Could you check a few things on this model? Use its own coordinates, in mm. A direction names the side the tool comes from. Round coordinates to 2 decimals unless told otherwise and drop trailing zeros. Loops run counter-clockwise (first coordinate to the right, second up) from the corner with the lowest first, then second, coordinate; pieces in that order, holes last. Notation, with made-up numbers: (-3, 66.5) - (32, 66.5) arc R37 ccw to (32, 104.5) - close; hole circle Ø5 at (50.25, -21). An arc over 180 degrees is marked (long way). Put each result on its own line as item: value. Start each with the question number.
from build123d import *

# Parameters (mm, degrees)
CROQUIS1_R              = 13
CROQUIS1_R_2            = 6
SALIENTE_EXTRUIR1_DEPTH = 10
CROQUIS2_W              = 30
CROQUIS2_H              = 15
SALIENTE_EXTRUIR2_DEPTH = 5
CROQUIS3_W              = 30
CROQUIS3_H              = 5
SALIENTE_EXTRUIR3_DEPTH = 20
CROQUIS4_R              = 5
CORTAR_EXTRUIR1_DEPTH   = 20
REDONDEO1_R             = 1
REDONDEO2_R             = 1
REDONDEO3_R             = 3
CROQUIS5_R              = 13
CROQUIS5_R_2            = 6
SALIENTE_EXTRUIR4_DEPTH = 5
CROQUIS6_R              = 20
CROQUIS6_R_2            = 13
SALIENTE_EXTRUIR5_DEPTH = 3
REDONDEO4_R             = 3


with BuildPart() as part:
    # Croquis1 → Saliente-Extruir1 (new body)
    with BuildSketch(Plane(origin=(0, 0, 0), x_dir=(1, 0, 0), z_dir=(0, 1, 0))):
        Polygon((-109.095, 0), (109.095, 0), (109.095, 29.37), (59.500415879, 165.63), (50.697846821, 170.712165615), (15.697846821, 170.712165615), (3.225, 157.21), (-64.095, 37.77), (-76.489816261, 30.39), (-103.085, 30.39), (-109.095, 22), align=None)
        with Locations(Location((33.197846821, 134.63, 0), (0, 0, 270))):
            Circle(CROQUIS1_R, mode=Mode.SUBTRACT)
        with Locations(Location((-64.095, 18, 0), (0, 0, 270))):
            Circle(CROQUIS1_R_2, mode=Mode.SUBTRACT)
        with Locations(Location((80.805, 18, 0), (0, 0, 270))):
            Circle(CROQUIS1_R_2, mode=Mode.SUBTRACT)
        with BuildLine():
            Line((-34.959241143, 24.905539046), (-16.329241143, 24.905539046))
            ThreePointArc((-16.329241143, 24.905539046), (-14.915027581, 25.491325484), (-14.329241143, 26.905539046))
            Line((-14.329241143, 26.905539046), (-14.329241143, 64.805539046))
            ThreePointArc((-14.329241143, 64.805539046), (-14.915027581, 66.219752609), (-16.329241143, 66.805539046))
            Line((-16.329241143, 66.805539046), (-28.864540605, 66.805539046))
            ThreePointArc((-28.864540605, 66.805539046), (-29.864540605, 66.537589854), (-30.596591412, 65.805539046))
            Line((-30.596591412, 65.805539046), (-45.124461509, 40.642529914))
            ThreePointArc((-45.124461509, 40.642529914), (-45.275154746, 38.967789325), (-44.095, 37.77))
            ThreePointArc((-44.095, 37.77), (-38.917486541, 33.735802046), (-36.959241143, 27.471085475))
            Line((-36.959241143, 27.471085475), (-36.959241143, 26.905539046))
            ThreePointArc((-36.959241143, 26.905539046), (-36.373454706, 25.491325484), (-34.959241143, 24.905539046))
        make_face(mode=Mode.SUBTRACT)
        with BuildLine():
            Line((70.518843068, 107.928122629), (93.592402069, 44.534040287))
            ThreePointArc((93.592402069, 44.534040287), (93.351320916, 42.702847127), (91.713016828, 41.85))
            Line((91.713016828, 41.85), (87.853935228, 41.85))
            ThreePointArc((87.853935228, 41.85), (86.557059698, 42.32746466), (85.879396403, 43.53188614))
            ThreePointArc((85.879396403, 43.53188614), (74.558636842, 45.862576394), (63.719312841, 41.85))
            ThreePointArc((63.719312841, 41.85), (62.305099279, 42.435786438), (61.719312841, 43.85))
            Line((61.719312841, 43.85), (61.719312841, 58.5))
            ThreePointArc((61.719312841, 58.5), (60.302618614, 70.31788476), (56.132816833, 81.466076355))
            Line((56.132816833, 81.466076355), (47.469675424, 99.515111912))
            ThreePointArc((47.469675424, 99.515111912), (47.413687511, 101.118061517), (48.553338923, 102.246678699))
            ThreePointArc((48.553338923, 102.246678699), (59.00154122, 103.684084154), (68.023190025, 109.146768338))
            ThreePointArc((68.023190025, 109.146768338), (69.517034466, 109.041263258), (70.518843068, 107.928122629))
        make_face(mode=Mode.SUBTRACT)
    extrude(amount=SALIENTE_EXTRUIR1_DEPTH)

    # Croquis2 → Saliente-Extruir2 (add)
    with BuildSketch(Plane(origin=(0, 10, 0), x_dir=(1, 0, 0), z_dir=(0, 1, 0))):
        with Locations((-29.095, 7.5)):
            Rectangle(CROQUIS2_W, CROQUIS2_H)
        with Locations((45.805, 7.5)):
            Rectangle(CROQUIS2_W, CROQUIS2_H)
    extrude(amount=SALIENTE_EXTRUIR2_DEPTH)

    # Croquis3 → Saliente-Extruir3 (add)
    with BuildSketch(Plane(origin=(0, 15, 0), x_dir=(1, 0, 0), z_dir=(0, 1, 0))):
        with Locations((-29.095, 2.5)):
            Rectangle(CROQUIS3_W, CROQUIS3_H)
        with Locations((45.805, 2.5)):
            Rectangle(CROQUIS3_W, CROQUIS3_H)
    extrude(amount=SALIENTE_EXTRUIR3_DEPTH)

    # Croquis4 → Cortar-Extruir1 (cut)
    with BuildSketch(Plane(origin=(0, 0, -5), x_dir=(-1, 0, 0), z_dir=(0, 0, -1))):
        with Locations((-45.805, 28)):
            Circle(CROQUIS4_R)
        with Locations((29.095, 28)):
            Circle(CROQUIS4_R)
    extrude(amount=-CORTAR_EXTRUIR1_DEPTH, mode=Mode.SUBTRACT)

    # Redondeo1
    redondeo1_edges = [part.edges().sort_by_distance(p)[0] for p in [
        (-14.095, 10, -7.5),
        (-44.095, 10, -7.5),
        (60.805, 10, -7.5),
        (30.805, 10, -7.5),
    ]]
    fillet(redondeo1_edges, radius=REDONDEO1_R)

    # Redondeo2
    redondeo2_edges = [part.edges().sort_by_distance(p)[0] for p in [
        (45.805, 10, -15),
        (-29.095, 10, -15),
    ]]
    fillet(redondeo2_edges, radius=REDONDEO2_R)

    # Redondeo3
    redondeo3_edges = [part.edges().sort_by_distance(p)[0] for p in [
        (-29.095, 15, -5),
        (45.805, 15, -5),
    ]]
    fillet(redondeo3_edges, radius=REDONDEO3_R)

    # Croquis5 → Saliente-Extruir4 (add)
    with BuildSketch(Plane.XZ):
        with Locations(Location((33.197846821, -134.63, 0), (0, 0, 270))):
            Circle(CROQUIS5_R)
        with Locations(Location((33.197846821, -134.63, 0), (0, 0, 270))):
            Circle(CROQUIS5_R_2, mode=Mode.SUBTRACT)
    extrude(amount=-SALIENTE_EXTRUIR4_DEPTH)

    # Croquis6 → Saliente-Extruir5 (add)
    with BuildSketch(Plane(origin=(0, 10, 0), x_dir=(1, 0, 0), z_dir=(0, 1, 0))):
        with Locations(Location((33.197846821, 134.63, 0), (0, 0, 270))):
            Circle(CROQUIS6_R)
        with Locations(Location((33.197846821, 134.63, 0), (0, 0, 90))):
            Circle(CROQUIS6_R_2, mode=Mode.SUBTRACT)
    extrude(amount=SALIENTE_EXTRUIR5_DEPTH)

    # Redondeo4
    redondeo4_edges = [part.edges().sort_by_distance(p)[0] for p in [
        (33.197846821, 13, -154.63),
    ]]
    fillet(redondeo4_edges, radius=REDONDEO4_R - 0.0001)  # a hair under: the kernel refuses the full size


solid = part.part
Item 1: Suppose I cut it at C-C, the plane z = -94.5. List the corners of the cut face in (x, y) for me.
Item 2: I need wall thicknesses on line 1 (X direction, y = 6.5, z = -18) (3 decimals); line 2 (Y direction, x = 6, z = -67); line 3 (Z direction, x = -22.5, y = 22). Which ranges of each line are inside material? Lowest first, please. Write a range as from..to.
Item 3: Suppose I cut it at A-A, the plane z = -54.5. List the corners of the cut face in (x, y) for me.
Item 4: On a 3-axis mill with a long thin cutter (end or side, diameter ignored), from which of +Z, -Z, +X, -X, +Y, -Y can I reach the whole of each face in a straight line? I mean faces 5 (the face through (-38.97, 4.93, -33.81)), 6 (the face through (30.805, 20, -4)), 7 (the face through (30, 5, -140)), 8 (the face through (-14.095, 20, -4)), 9 (the face through (-24.1, 28.2, -2.5)). Say none if no direction works.
Item 5: Suppose I cut it at B-B, the plane y = 28. List the corners of the cut face in (x, z) for me (3 decimals).
Item 6: Thinking about a two-plate mould opening in X: for faces 1 (the face through (61.719, 5, -51)), 2 (the face through (74.722, 4.93, -45.874)), 3 (the face through (9.549, 4.93, -164.056)), 4 (the face through (-29, 15, -12)), which applies, released by +X, released by -X, zero draft, split by the parting line, or undercut?
Item 7: Will these pins go through, and if not, where does the flat tip stop? P1, Ø5, axis at x = -96, y = 3, coming from the -Z side; P2, Ø8, axis at y = 6.5, z = -52, coming from the -X side; P3, Ø14, axis at x = 33.2, z = -134.63, coming from the +Y side; P4, Ø3, axis at x = -15, z = -19, coming from the -Y side.
Item 8: Suppose I cut it at D-D, the plane x = -91. List the corners of the cut face in (y, z) for me.
Numbers:
1. outline: (-32.12, 0) - (49.88, 0) - (49.88, 10) - (-32.12, 10) - close; (75.41, 0) - (85.39, 0) - (85.39, 10) - (75.41, 10) - close
2. line 1: -109.095..-70.095, -58.095..74.805, 86.805..109.095
2. line 2: 0..10
2. line 3: -5..0
3. outline: (-54.67, 0) - (-37.12, 0) - (-37.12, 10) - (-54.67, 10) - close; (-14.33, 0) - (61.72, 0) - (61.72, 10) - (-14.33, 10) - close; (89.97, 0) - (99.95, 0) - (99.95, 10) - (89.97, 10) - close
4. face 5: +Y, -Y
4. face 6: +Z, +Y
4. face 7: +Y
4. face 8: +Z, -Z, +Y
4. face 9: +Z, -Z
5. outline: (-44.095, -5) - (-34.095, -5) - (-34.095, 0) - (-44.095, 0) - close; (-24.095, -5) - (-14.095, -5) - (-14.095, 0) - (-24.095, 0) - close; (30.805, -5) - (40.805, -5) - (40.805, 0) - (30.805, 0) - close; (50.805, -5) - (60.805, -5) - (60.805, 0) - (50.805, 0) - close
6. face 1: undercut
6. face 2: undercut
6. face 3: released by -X
6. face 4: zero draft
7. P1: z = -30.39
7. P2: x = -58.33
7. P3: y = 5
7. P4: y = 0
8. outline: (0, -30.39) - (10, -30.39) - (10, 0) - (0, 0) - close
